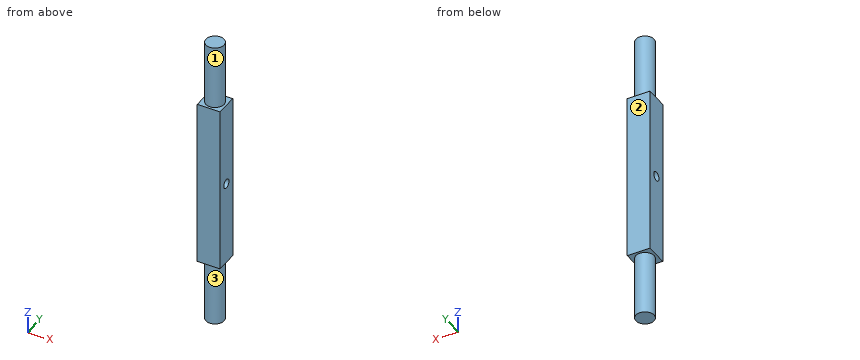
```python
from build123d import *

# Parameters (mm, degrees)
BOSS_EXTRUDE1_DEPTH      = 92.5
BOSS_EXTRUDE1_DEPTH_BACK = 92.5
SKETCH1_W                = 25
SKETCH1_H                = 25
SKETCH2_R                = 5
CUT_EXTRUDE1_DEPTH       = 100.026511602
SKETCH3_R                = 10
BOSS_EXTRUDE2_DEPTH      = 70
BOSS_EXTRUDE3_START      = 70
SKETCH4_R                = 10
BOSS_EXTRUDE3_DEPTH      = 70


with BuildPart() as part:
    # Sketch1 → Boss-Extrude1 (new, two sides: drawn at the far end of the back side and taken through both)
    with BuildSketch(Plane.XY.offset(-BOSS_EXTRUDE1_DEPTH_BACK)):
        with Locations((12.5, 12.5)):
            Rectangle(SKETCH1_W, SKETCH1_H)
    extrude(amount=BOSS_EXTRUDE1_DEPTH + BOSS_EXTRUDE1_DEPTH_BACK)

    # Sketch2 → Cut-Extrude1 (cut, through all)
    with BuildSketch(Plane(origin=(25, 0, 0), x_dir=(0, 0, -1), z_dir=(1, 0, 0))):
        with Locations((0, 12.5)):
            Circle(SKETCH2_R)
    extrude(amount=-CUT_EXTRUDE1_DEPTH, mode=Mode.SUBTRACT)

    # Sketch3 → Boss-Extrude2 (add)
    with BuildSketch(Plane.XY.offset(92.5)):
        with Locations((12.5, 12.5)):
            Circle(SKETCH3_R)
    extrude(amount=BOSS_EXTRUDE2_DEPTH)

    # Sketch4 → Boss-Extrude3 (add)
    with BuildSketch(Plane(origin=(0, 0, -92.5), x_dir=(-1, 0, 0), z_dir=(0, 0, -1)).offset(BOSS_EXTRUDE3_START)):
        with Locations(Location((-12.5, 12.5, 0), (0, 0, 180))):
            Circle(SKETCH4_R)
    extrude(amount=-BOSS_EXTRUDE3_DEPTH)


solid = part.part
```
Verification items for the finished model (mm, model axes). Face numbers are marked on the shaded views. A direction names the side the tool comes from. Coordinates: 2 decimals unless noted, no trailing zeros. Write each loop counter-clockwise with the first axis right and the second up, starting at its lowest first coordinate (ties: lowest second). Pieces come first, ordered by that corner, then holes. Notation, with made-up numbers: M 23.5,69 L 51.5,69 A14 ccw 51.5,93 Z; hole C 20,-18.5 d11. An arc over 180 degrees is marked long. Answer as a JSON object with one key per item and string values. Group by question number.
(1) Cross-section at C-C, the plane x = 12.5. Record the cut outline in (y, z).
(2) Cross-section at A-A, the plane y = 12.5. Record the cut outline in (x, z).
(3) Material ranges on line 1 (Y direction, x = 12.75, z = 0); line 2 (Z direction, x = 11, y = 8.25); line 3 (Z direction, x = 24, y = 13.25), recorded low to high.
(4) Tool access check on the marked faces 1, 2 and 3. Record the directions out of +Z, -Z, +X, -X, +Y, -Y that give a thin tool (end or side, any length) a straight path to the whole face; none if there is none.
(5) Cross-section at B-B, the plane z = 0. Record the cut outline in (x, y), and give its area (3 significant figures).
(6) Gauge pin test, flat ends, axial feed: pin 1 (4 mm diameter, centred on y = 11, z = 37, fed in from -X); pin 2 (8 mm diameter, centred on x = 10.5, z = 122, fed in from +Y). Record the tip position at first contact, or that the pin passes through.
Reply:
{
 "1": {"outline": "M 0,-92.5 L 2.5,-92.5 L 2.5,-162.5 L 22.5,-162.5 L 22.5,-92.5 L 25,-92.5 L 25,92.5 L 22.5,92.5 L 22.5,162.5 L 2.5,162.5 L 2.5,92.5 L 0,92.5 Z; hole C 12.5,0 d10"},
 "2": {"outline": "M 0,-92.5 L 2.5,-92.5 L 2.5,-162.5 L 22.5,-162.5 L 22.5,-92.5 L 25,-92.5 L 25,-5 L 0,-5 Z; M 0,5 L 25,5 L 25,92.5 L 22.5,92.5 L 22.5,162.5 L 2.5,162.5 L 2.5,92.5 L 0,92.5 Z"},
 "3": {"line 1": "0 to 7.5, 17.5 to 25", "line 2": "-162.5 to -2.63, 2.63 to 162.5", "line 3": "-92.5 to -4.94, 4.94 to 92.5"},
 "4": {"face 1": "+Z", "face 2": "+Z, -Z, +X, -X, +Y", "face 3": "-Z"},
 "5": {"outline": "M 0,0 L 25,0 L 25,7.5 L 0,7.5 Z; M 0,17.5 L 25,17.5 L 25,25 L 0,25 Z", "area": "375 mm²"},
 "6": {"pin 1": "x = 0", "pin 2": "y = 22.5"}
}
